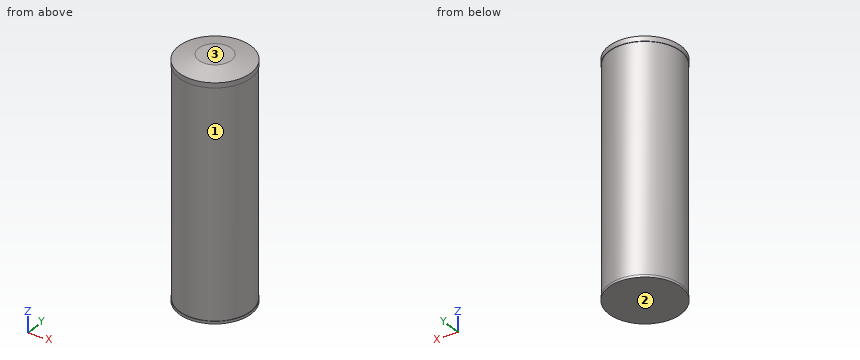
from build123d import *

# Parameters (mm, degrees)
F0_R     = 185.42
F1_DEPTH = 12.7
F2_R     = 182.88
F2_R_2   = 181.61
F3_DEPTH = 1181.1
F4_R     = 185.42
F5_DEPTH = 25.4
F6_SIZE2 = 25.39999
F6_SIZE  = 101.59999
F7_R     = 185.42
F7_R_2   = 182.88
F8_DEPTH = 25.4


# Not quite as in the source:
# - a fillet or chamfer is up to 0.001 mm smaller than in the source, because OpenCascade refuses the exact size


with BuildPart() as f1:
    # F0 (on Top) → F1 (new body)
    with BuildSketch(Plane.XY):
        Circle(F0_R)
    extrude(amount=F1_DEPTH)

    # F2 (on face) → F3 (join)
    with BuildSketch(Plane.XY.offset(12.7)):
        Circle(F2_R)
        Circle(F2_R_2, mode=Mode.SUBTRACT)
    extrude(amount=F3_DEPTH)

    # F4 (on face) → F5 (join)
    with BuildSketch(Plane.XY.offset(1193.8)):
        Circle(F4_R)
    extrude(amount=F5_DEPTH)

    # F6 (size 101.6 and 25.4 in the source; OpenCascade refuses exactly that, so slightly less here)
    f6_edges = [f1.edges().sort_by_distance(p)[0] for p in [
        (-185.42, 0, 1219.2),
    ]]
    f6_side = f1.faces().sort_by_distance((0, 0, 1219.2))[0]
    chamfer(f6_edges, length=F6_SIZE, length2=F6_SIZE2, reference=f6_side)

    # F7 (on face) → F8 (join)
    with BuildSketch(Plane(origin=(0, 0, 1193.8), x_dir=(1, 0, 0), z_dir=(0, 0, -1))):
        Circle(F7_R)
        Circle(F7_R_2, mode=Mode.SUBTRACT)
    extrude(amount=F8_DEPTH)


solid = f1.part
CAD build for the part. Positions are in the model's coordinates, mm. Face numbers are marked on the shaded views. Coordinates: 2 decimals unless noted, no trailing zeros. Order: outer loops, then holes, each group sorted by start corner. A loop starts at its lowest first (then second) coordinate and runs counter-clockwise, first axis right, second up.
Item 1: Drill centre lines: L1, parallel to Z at x = -11, y = -64.5; L2, parallel to Y at x = 0, z = 651; L3, parallel to X at y = 2.5, z = 898. Where is each one in solid material? Low to high.
Check sheet entries:
L1: z = 0 to 12.7, 1193.8 to 1219.2
L2: y = -182.88 to -181.61, 181.61 to 182.88
L3: x = -182.86 to -181.59, 181.59 to 182.86
Item 2: Two-plate mould, pull along Z, no slides. Class the marked faces 1, 2 and 3: +Z half, -Z half, draft (parallel to the pull), parting line (faces both ways), or undercut.
Check sheet entries:
face 1: undercut
face 2: -Z half
face 3: +Z half
Item 3: Band-saw the part on A-A on y = 0. List the corners of the cut face in (x, z).
Check sheet entries:
outline: (-185.42, 0) - (185.42, 0) - (185.42, 12.7) - (182.88, 12.7) - (182.88, 1168.4) - (185.42, 1168.4) - (185.42, 1193.8) - (83.82, 1219.2) - (-83.82, 1219.2) - (-185.42, 1193.8) - (-185.42, 1168.4) - (-182.88, 1168.4) - (-182.88, 12.7) - (-185.42, 12.7) - close; hole (-181.61, 12.7) - (181.61, 12.7) - (181.61, 1193.8) - (-181.61, 1193.8) - close
Item 4: Band-saw the part on C-C on z = 641.5. List the corners of the cut face in (x, y).
Check sheet entries:
outline: circle Ø365.76 at (0, 0); hole circle Ø363.22 at (0, 0)
Item 5: Pin check, flat tips, straight feed: pin 1 Ø8 at (x, y) = (-131, -81.5) entering from +Z; pin 2 Ø5 at (x, z) = (-5.5, 465.5) entering from -Y; pin 3 Ø8 at (x, z) = (-118, 461.5) entering from -Y. Stop position of each tip, or through.
Check sheet entries:
pin 1: stops at z = 1202.58
pin 2: stops at y = -182.86
pin 3: stops at y = -143
